Read the model definition and answer for the solid it produces. Units are mm, in the model's axes. Face numbers are marked on the shaded views. A direction names the side the tool comes from. Coordinates: 2 decimals unless noted, no trailing zeros. Write each loop counter-clockwise with the first axis right and the second up, starting at its lowest first coordinate (ties: lowest second). Pieces come first, ordered by that corner, then holes. Notation, with made-up numbers: (56.5, 38) -> (61.5, 38) arc R27 cw to (61.5, 63) -> close; hole circle Ø5 at (-30.5, -15.75). An arc over 180 degrees is marked (long way). One line per item, written item: value. Start each with the question number.
1. Find section C-C, the plane y = 6.25. Write down the section's boundary in (x, z), and give its area (3 significant figures).
2. Find section A-A, the plane z = 0. Write down the section's boundary in (x, y).
3. Given P1, Ø2, axis at x = 16.5, z = -9.5, coming from the +Y side; P2, Ø7.5, axis at x = 0, z = 19, coming from the -Y side; P3, Ø3, axis at x = -0.5, z = 18, coming from the +Y side; P4, Ø1, axis at x = -15.5, y = 3, coming from the +Z side, each flat-ended and moving along its own axis, determine where each tip first touches the part or whether it passes through.
4. For the marked faces 1 and 2, determine the directions among +Z, -Z, +X, -X, +Y, -Y from which every point of the face is accessible in a straight line to the end or side of a thin tool.
5. Find section B-B, the plane x = 0. State how many separate pieces and enclosed holes the cut face has, and give its area (3 significant figures).
6. Consider line 1 along X through (y, z) = (4.3, 0); line 2 along Y through (x, z) = (-7, -4); line 3 along Y through (x, z) = (17.5, -2.5). Determine where each line is inside the solid, lowest interval first.
7. For a pull along X with two mould halves and no side action, classify the marked faces 3, 4 and 5 as pulls with the +X half, pulls with the -X half, needs draft (parallel to the pull), parting line crosses it, or undercut.
```python
from build123d import *

# Parameters (mm, degrees)
CHANFREIN2_SIZE                                    = 0.5
CHANFREIN2_SIZE2                                   = 0.288675135
CHANFREIN3_SIZE                                    = 0.5
CHANFREIN4_SIZE                                    = 0.5
CHANFREIN5_SIZE                                    = 0.5
CHAMBRAGE_POUR_VIS_T_TE_HEXAGONALE_M31_D           = 3.4
CHAMBRAGE_POUR_VIS_T_TE_HEXAGONALE_M31_CBORE_D     = 6.5
CHAMBRAGE_POUR_VIS_T_TE_HEXAGONALE_M31_CBORE_DEPTH = 3
R_P_TITION_CIRCULAIRE1_COUNT                       = 3


with BuildPart() as part:
    # Esquisse1 → Révolution1 (revolve)
    with BuildSketch(Plane.XY, mode=Mode.PRIVATE) as r_volution1_sk:
        Polygon((11.75, 0), (15, 0), (15, 3), (23, 3), (23, 8), (6, 8), (6, 2), (11.75, 2), align=None)
    revolve(r_volution1_sk.sketch.rotate(Axis((0, 0, 0), (0, 1, 0)), 90), axis=Axis((0, 0, 0), (0, 1, 0)))  # turned: the seam where the file's is

    # Chanfrein2
    chanfrein2_edges = [part.edges().sort_by_distance(p)[0] for p in [
        (0, 0, 15),
    ]]
    chanfrein2_side = [part.faces().sort_by_distance(p)[0] for p in [
        (0, 1.5, 15),
    ]]
    chamfer(chanfrein2_edges, length=CHANFREIN2_SIZE, length2=CHANFREIN2_SIZE2, reference=chanfrein2_side[0])

    # Chanfrein3
    chanfrein3_edges = [part.edges().sort_by_distance(p)[0] for p in [
        (0, 8, 6),
    ]]
    chamfer(chanfrein3_edges, length=CHANFREIN3_SIZE)

    # Chanfrein4
    chanfrein4_edges = [part.edges().sort_by_distance(p)[0] for p in [
        (0, 2, 6),
    ]]
    chamfer(chanfrein4_edges, length=CHANFREIN4_SIZE)

    # Chanfrein5
    chanfrein5_edges = [part.edges().sort_by_distance(p)[0] for p in [
        (0, 8, 23),
    ]]
    chamfer(chanfrein5_edges, length=CHANFREIN5_SIZE)

    # Chambrage pour vis à tête hexagonale M31 (through all)
    with Locations(Plane(origin=(0, 8, 0), x_dir=(-1, 0, 0), z_dir=(0, 1, 0))):
        with Locations((0, 19)):
            chambrage_pour_vis_t_te_hexagonale_m31 = CounterBoreHole(CHAMBRAGE_POUR_VIS_T_TE_HEXAGONALE_M31_D / 2, CHAMBRAGE_POUR_VIS_T_TE_HEXAGONALE_M31_CBORE_D / 2, CHAMBRAGE_POUR_VIS_T_TE_HEXAGONALE_M31_CBORE_DEPTH)

    # Répétition circulaire1: Chambrage pour vis à tête hexagonale M31 ×3 about axis
    r_p_tition_circulaire1_axis = Axis((0, 0, 0), (0, 1, 0))
    for i in range(1, R_P_TITION_CIRCULAIRE1_COUNT):
        add(chambrage_pour_vis_t_te_hexagonale_m31.rotate(r_p_tition_circulaire1_axis, i * 360 / R_P_TITION_CIRCULAIRE1_COUNT), mode=Mode.SUBTRACT)


solid = part.part
```
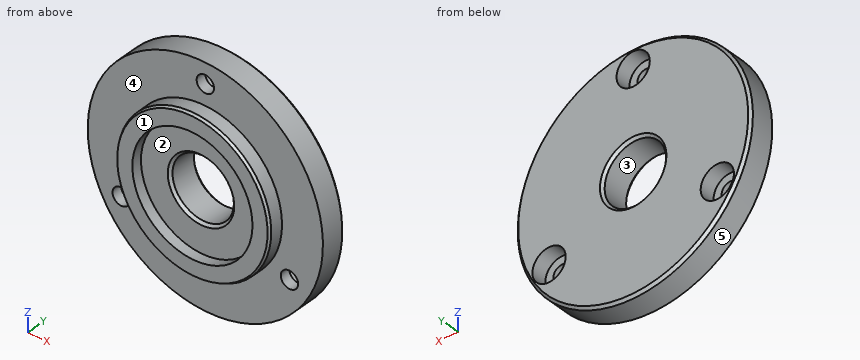
Answer block:
1. outline: circle Ø46 at (0, 0); hole circle Ø6.5 at (-16.45, -9.5); hole circle Ø12 at (0, 0); hole circle Ø6.5 at (0, 19); hole circle Ø6.5 at (16.45, -9.5)
1. area: 1,450 mm2
2. outline: (-23, 3) -> (-15, 3) -> (-15, 0.5) -> (-14.71, 0) -> (-11.75, 0) -> (-11.75, 2) -> (-6.5, 2) -> (-6, 2.5) -> (-6, 7.5) -> (-6.5, 8) -> (-22.5, 8) -> (-23, 7.5) -> close; (6, 2.5) -> (6.5, 2) -> (11.75, 2) -> (11.75, 0) -> (14.71, 0) -> (15, 0.5) -> (15, 3) -> (23, 3) -> (23, 7.5) -> (22.5, 8) -> (6.5, 8) -> (6, 7.5) -> close
3. P1: passes through
3. P2: stops at y = 3
3. P3: stops at y = 5
3. P4: stops at z = 17.44
4. face 1: +Z, -Z, +X, -X, -Y
4. face 2: -Y
5. separate pieces: 3
5. enclosed holes: 0
5. area: 174 mm2
6. line 1: x = -23 to -6, 6 to 23
6. line 2: y = 2 to 8
6. line 3: y = 3 to 8
7. face 3: undercut
7. face 4: needs draft
7. face 5: parting line crosses it
